Input: part model. Units: mm. Frame: model coordinates. A direction names the side the tool comes from. Coordinates: 2 decimals unless noted, no trailing zeros. Write each loop counter-clockwise with the first axis right and the second up, starting at its lowest first coordinate (ties: lowest second). Pieces come first, ordered by that corner, then holes.
1) Set-up query: faces 5 (the flat face through (-26, 7.5, 17)), 6 (the flat face through (17, 15, 17)), 7 (the flat face through (0, -25, 17)). Return all of +Z, -Z, +X, -X, +Y, -Y with unobstructed straight access to the full face (end or side cutting, diameter ignored); none if empty.
2) Section query D-D (z = 29). Output: boundary loops of the cut face in (x, y), then the cut area to 3 significant figures.
3) Section query B-B (y = 0). Output: boundary loops of the cut face in (x, z).
4) Section query C-C (x = -23). Output: boundary loops of the cut face in (y, z).
5) Line query: L1, parallel to Y at x = 0, z = 3; L2, parallel to X at y = -12, z = 13.5; L3, parallel to X at y = -4.5, z = 12. Output: solid intervals per line, ascending.
6) Pin query (flat end, axial travel): pin 1 Ø12 at (y, z) = (14, 5.5) entering from -X; pin 2 Ø15.5 at (y, z) = (17, 9) entering from +X; pin 3 Ø12 at (x, z) = (-22.5, 29) entering from +Y; pin 4 Ø7 at (x, y) = (0, 0) entering from +Z. Return the tip coordinate at first contact, or that it passes through.
7) Draft query along X for faces 1 (the flat face through (-30, -9, 17)), 2 (the cylindrical face through (-6, 0, 17)), 3 (the cylindrical face through (25.395, -8.522, 17.197)), 4 (the flat face through (26, 7.5, 17)). Return one class per face: pulls with the +X half, pulls with the -X half, needs draft (parallel to the pull), parting line crosses it, or undercut.
8) Section query A-A (z = 15). Output: boundary loops of the cut face in (x, y).
from build123d import *

# Parameters (mm, degrees)
SKETCH_R     = 6
PAD_DEPTH    = 35
SKETCH001_R  = 3.25
POCKET_DEPTH = 32.501


with BuildPart() as part:
    # Sketch → Pad (new body)
    with BuildSketch(Plane.XY):
        Polygon((-17, 21.625642), (17, 21.625642), (17, 7.5), (30, 7.5), (30, -25), (-30, -25), (-30, 7.5), (-17, 7.5), align=None)
        Circle(SKETCH_R, mode=Mode.SUBTRACT)
    extrude(amount=PAD_DEPTH)

    # Sketch001 (on Face7 of Pad) → Pocket (cut, through all)
    with BuildSketch(Plane(origin=(0, 7.5, 0), x_dir=(-1, 0, 0), z_dir=(0, 1, 0))):
        with Locations((-23, 15)):
            Circle(SKETCH001_R)
        with Locations((23, 15)):
            Circle(SKETCH001_R)
    extrude(amount=-POCKET_DEPTH, mode=Mode.SUBTRACT)


solid = part.part
Answer:
1. face 5: +Z, -Z, -X, +Y
1. face 6: +Z, -Z, +X, +Y
1. face 7: +Z, -Z, +X, -X, -Y
2. outline: (-30, -25) - (30, -25) - (30, 7.5) - (17, 7.5) - (17, 21.63) - (-17, 21.63) - (-17, 7.5) - (-30, 7.5) - close; hole circle Ø12 at (0, 0)
2. area: 2,320 mm2
3. outline: (-30, 0) - (-6, 0) - (-6, 35) - (-30, 35) - close; (6, 0) - (30, 0) - (30, 35) - (6, 35) - close; hole circle Ø6.5 at (-23, 15); hole circle Ø6.5 at (23, 15)
4. outline: (-25, 0) - (7.5, 0) - (7.5, 11.75) - (-25, 11.75) - close; (-25, 18.25) - (7.5, 18.25) - (7.5, 35) - (-25, 35) - close
5. L1: y = -25 to -6, 6 to 21.63
5. L2: x = -30 to -25.88, -20.12 to 20.12, 25.88 to 30
5. L3: x = -30 to -24.25, -21.75 to -3.97, 3.97 to 21.75, 24.25 to 30
6. pin 1: stops at x = -17
6. pin 2: stops at x = 17
6. pin 3: stops at y = 21.63
6. pin 4: passes through
7. face 1: pulls with the -X half
7. face 2: undercut
7. face 3: undercut
7. face 4: needs draft
8. outline: (-30, -25) - (-26.25, -25) - (-26.25, 7.5) - (-30, 7.5) - close; (-19.75, -25) - (19.75, -25) - (19.75, 7.5) - (17, 7.5) - (17, 21.63) - (-17, 21.63) - (-17, 7.5) - (-19.75, 7.5) - close; (26.25, -25) - (30, -25) - (30, 7.5) - (26.25, 7.5) - close; hole circle Ø12 at (0, 0)
